from build123d import *

# Parameters (mm, degrees)
BOSS_EXTRUDE1_DEPTH = 15.5
CUT_EXTRUDE1_DEPTH  = 81.5


with BuildPart() as part:
    # Sketch1 → Boss-Extrude1 (new body)
    with BuildSketch(Plane.XY):
        Polygon((-10.229681979, -19.726325088), (-70.229681979, -19.726325088), (-70.229681979, -29.913296732), (-76.585734932, -29.913296732), (-76.585734932, -30.976616664), (-70.229681979, -30.976616664), (-70.229681979, -32.376325088), (-68.814681979, -32.376325088), (-68.029681979, -29.801896387), (-67.244681979, -32.376325088), (-66.459681979, -29.801896387), (-65.674681979, -32.376325088), (-64.889681979, -29.801896387), (-64.104681979, -32.376325088), (-63.319681979, -29.801896387), (-62.534681979, -32.376325088), (-61.749681979, -29.801896387), (-60.964681979, -32.376325088), (-60.179681979, -29.801896387), (-59.394681979, -32.376325088), (-58.609681979, -29.801896387), (-57.824681979, -32.376325088), (-57.039681979, -29.801896387), (-56.254681979, -32.376325088), (-55.469681979, -29.801896387), (-54.684681979, -32.376325088), (-53.899681979, -29.801896387), (-53.114681979, -32.376325088), (-52.329681979, -29.801896387), (-51.544681979, -32.376325088), (-50.759681979, -29.801896387), (-49.974681979, -32.376325088), (-49.189681979, -29.801896387), (-48.404681979, -32.376325088), (-47.619681979, -29.801896387), (-46.834681979, -32.376325088), (-46.049681979, -29.801896387), (-45.264681979, -32.376325088), (-44.479681979, -29.801896387), (-43.694681979, -32.376325088), (-42.909681979, -29.801896387), (-42.124681979, -32.376325088), (-41.339681979, -29.801896387), (-40.554681979, -32.376325088), (-39.769681979, -29.801896387), (-38.984681979, -32.376325088), (-38.199681979, -29.801896387), (-37.414681979, -32.376325088), (-36.629681979, -29.801896387), (-35.844681979, -32.376325088), (-35.059681979, -29.801896387), (-34.274681979, -32.376325088), (-33.489681979, -29.801896387), (-32.704681979, -32.376325088), (-31.919681979, -29.801896387), (-31.134681979, -32.376325088), (-30.349681979, -29.801896387), (-29.564681979, -32.376325088), (-28.779681979, -29.801896387), (-27.994681979, -32.376325088), (-27.209681979, -29.801896387), (-26.424681979, -32.376325088), (-25.639681979, -29.801896387), (-24.854681979, -32.376325088), (-24.069681979, -29.801896387), (-23.284681979, -32.376325088), (-22.499681979, -29.801896387), (-21.714681979, -32.376325088), (-20.929681979, -29.801896387), (-20.144681979, -32.376325088), (-19.359681979, -29.801896387), (-18.574681979, -32.376325088), (-17.789681979, -29.801896387), (-17.004681979, -32.376325088), (-16.219681979, -29.801896387), (-15.434681979, -32.376325088), (-14.649681979, -29.801896387), (-13.864681979, -32.376325088), (-13.079681979, -29.801896387), (-12.294681979, -32.376325088), (-11.509681979, -29.801896387), (-10.724681979, -32.376325088), (-10.229681979, -32.376325088), align=None)
    extrude(amount=BOSS_EXTRUDE1_DEPTH)

    # Sketch2 → Cut-Extrude1 (cut)
    with BuildSketch(Plane.ZY.offset(70.229681979)):
        with BuildLine():
            Line((6.05, -23.826325088), (5, -23.826325088))
            ThreePointArc((5, -23.826325088), (3.585786438, -24.412111526), (3, -25.826325088))
            Line((3, -25.826325088), (3, -28.026325088))
            Line((3, -28.026325088), (12.5, -28.026325088))
            Line((12.5, -28.026325088), (12.5, -25.826325088))
            ThreePointArc((12.5, -25.826325088), (11.914213562, -24.412111526), (10.5, -23.826325088))
            Line((10.5, -23.826325088), (9.45, -23.826325088))
            Line((9.45, -23.826325088), (9.45, -19.726325088))
            Line((9.45, -19.726325088), (6.05, -19.726325088))
            Line((6.05, -19.726325088), (6.05, -23.826325088))
        make_face()
    extrude(amount=-CUT_EXTRUDE1_DEPTH, mode=Mode.SUBTRACT)


solid = part.part
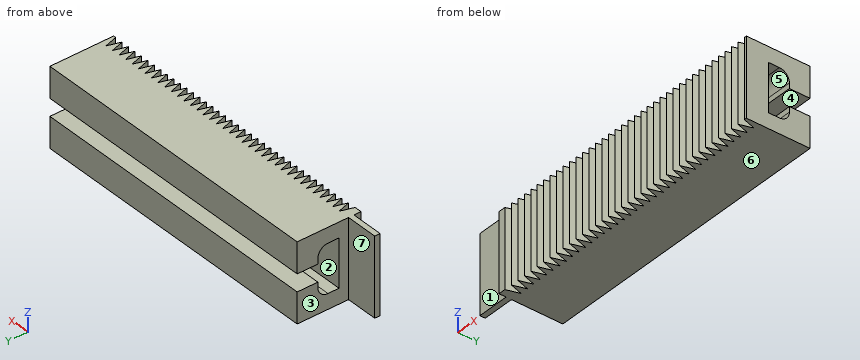
The listing builds one solid part. Answer for the finished solid, in the listing's coordinates (mm). Face numbers are marked on the shaded views. A direction names the side the tool comes from. Give positions to 0.01 mm unless a question says otherwise; leave off trailing zeros. Order: outer loops, then holes, each group sorted by start corner. A loop starts at its lowest first (then second) coordinate and runs counter-clockwise, first axis right, second up. Notation, with made-up numbers: (45, 54) -> (99, 54) arc R15 ccw to (99, 69) -> close; hole circle Ø3 at (-13.75, 22.25). An arc over 180 degrees is marked (long way). Put each result on its own line as item: value.
Item 1: For a pull along Y with two mould halves and no side action, classify the marked faces 5, 6 and 7 as released by +Y, released by -Y, zero draft, split by the parting line, or undercut.
Established:
face 5: undercut
face 6: zero draft
face 7: released by +Y
Item 2: A cutting plane is placed at B-B on y = -29. Give the vertices of the cut face in (x, z).
Established:
outline: (-70.23, 0) -> (-10.23, 0) -> (-10.23, 15.5) -> (-70.23, 15.5) -> close
Item 3: Straight lines are drawn through the part: line 1 (Z direction, x = -13, y = -22.75); line 2 (X direction, y = -25.5, z = 0.75); line 3 (Z direction, x = -22.5, y = -24.25). For each, find the intervals that lie inside material, in ascending order.
Established:
line 1: z = 0 to 6.05, 9.45 to 15.5
line 2: x = -70.23 to -10.23
line 3: z = 0 to 3.77, 11.73 to 15.5
Item 4: A cutting plane is placed at A-A on y = -26.5. Give the vertices of the cut face in (x, z).
Established:
outline: (-70.23, 0) -> (-10.23, 0) -> (-10.23, 3) -> (-70.23, 3) -> close; (-70.23, 12.5) -> (-10.23, 12.5) -> (-10.23, 15.5) -> (-70.23, 15.5) -> close
Item 5: For the marked faces 1, 2, 3 and 4, determine the directions among +Z, -Z, +X, -X, +Y, -Y from which every point of the face is accessible in a straight line to the end or side of a thin tool.
Established:
face 1: +Z, -Z, -X, -Y
face 2: +X, -X
face 3: +Z, -Z, -X, +Y
face 4: +X, -X, +Y
Item 6: Given P1, Ø5, axis at x = -74, z = 5, coming from the +Y side; P2, Ø1.5, axis at x = -61.5, z = 4.5, coming from the -Y side; P3, Ø7, axis at x = -75, z = 6, coming from the -Y side, each flat-ended and moving along its own axis, determine where each tip first touches the part or whether it passes through.
Established:
P1: stops at y = -29.91
P2: stops at y = -32.38
P3: stops at y = -30.98
